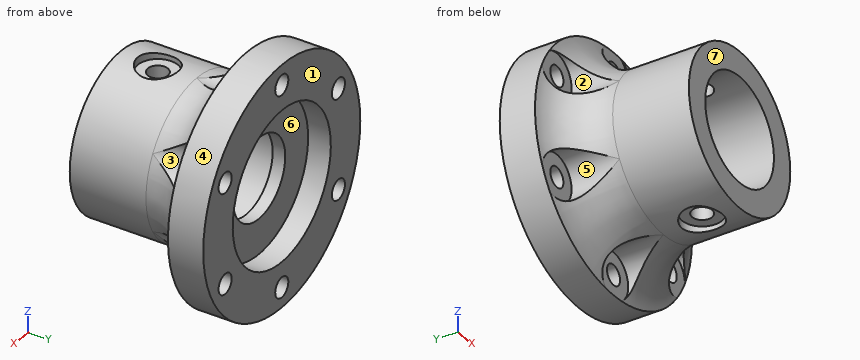
from build123d import *

# Parameters (mm, degrees)
SKETCH_1_R          = 15.5
SKETCH_1_R_2        = 10.5
EXTRUDE_1_DEPTH     = 25
SKETCH_3_R          = 24
EXTRUDE_2_DEPTH     = 7
FILLET_1_R          = 10
SKETCH_5_R          = 15
CUT_EXTRUDE_3_DEPTH = 4.5
SKETCH_6_R          = 8
CUT_EXTRUDE_4_DEPTH = 44.683520920365446
SKETCH_7_R          = 2.0000000000000018
SKETCH_7_R_2        = 2.0000000000000036
SKETCH_7_R_3        = 2.0000000000000004
SKETCH_7_R_4        = 2.0000000000000013
SKETCH_7_R_5        = 2.000000000000003
SKETCH_7_R_6        = 2
CUT_EXTRUDE_5_DEPTH = 47.64761515876246
CUT_EXTRUDE_START   = -7
SKETCH_8_R          = 4.500000000000001
SKETCH_8_R_2        = 4.500000000000002
SKETCH_8_R_3        = 4.5000000000000036
SKETCH_8_R_4        = 4.499999999999999
CUT_EXTRUDE_6_DEPTH = 10
SKETCH_9_R          = 2
CUT_EXTRUDE_7_DEPTH = 20
CUT_EXTRUDE_START_2 = -14
SKETCH_11_R         = 4
CUT_EXTRUDE_8_DEPTH = 40
CUT_EXTRUDE_START_3 = 54
SKETCH_12_R         = 4
CUT_EXTRUDE_9_DEPTH = 40


with BuildPart() as part:
    # Эскиз1 → Вытянуть1 (new body)
    with BuildSketch(Plane(origin=(0, 0, 0), x_dir=(1, 0, 0), z_dir=(0, 1, 0))):
        with Locations(Location((0, 0, 0), (0, 0, 270))):
            Circle(SKETCH_1_R)
        with Locations(Location((0, 0, 0), (0, 0, 270))):
            Circle(SKETCH_1_R_2, mode=Mode.SUBTRACT)
    extrude(amount=EXTRUDE_1_DEPTH)

    # Эскиз3 → Вытянуть2 (add)
    with BuildSketch(Plane(origin=(0, 25, 0), x_dir=(1, 0, 0), z_dir=(0, 1, 0))):
        with Locations(Location((0, 0, 0), (0, 0, 270))):
            Circle(SKETCH_3_R)
    extrude(amount=EXTRUDE_2_DEPTH)

    # Скругление1
    # the kernel refuses this fillet: 10 mm, written as the material it adds along each edge
    with BuildSketch(Plane(origin=(0, 25, 0), x_dir=(-1.8e-16, 0, 1), z_dir=(-1, 0, -1.8e-16))) as fillet_1_piece_1:
        with BuildLine():
            CenterArc((25.5, -9.886859966642819), FILLET_1_R, 98.62692655867845, 81.37307344132155)
            Line((15.5, -9.886859966642819), (15.3, -9.886859966642819))
            Line((15.3, -9.886859966642819), (15.3, 0))
            Line((15.3, 0), (15.5, 0.1999999999999993))
            ThreePointArc((15.5, 0.1999999999999993), (19.750000000000014, 0.1999999999999993), (23.970000000000034, 0.19773719933263223))
            Line((23.970000000000034, 0.19773719933263223), (24.000000000000032, -2.2027e-13))
        make_face()
    revolve(axis=Axis((0, 25, 0), (0, 1, 0)))

    # Эскиз5 → Вытянуть3 (cut)
    with BuildSketch(Plane(origin=(0, 32, 0), x_dir=(1, 0, 0), z_dir=(0, 1, 0))):
        with Locations(Location((0, 0, 0), (0, 0, 270))):
            Circle(SKETCH_5_R)
    extrude(amount=-CUT_EXTRUDE_3_DEPTH, mode=Mode.SUBTRACT)

    # Эскиз6 → Вытянуть4 (cut, through all)
    with BuildSketch(Plane(origin=(0, 27.5, 0), x_dir=(1, 0, 0), z_dir=(0, 1, 0))):
        with Locations(Location((0, 0, 0), (0, 0, 270))):
            Circle(SKETCH_6_R)
    extrude(amount=-CUT_EXTRUDE_4_DEPTH, mode=Mode.SUBTRACT)

    # Эскиз7 → Вытянуть5 (cut, through all)
    with BuildSketch(Plane(origin=(0, 32, 0), x_dir=(1, 0, 0), z_dir=(0, 1, 0))):
        with Locations(Location((0, -20, 0), (0, 0, 270))):
            Circle(SKETCH_7_R)
        with Locations(Location((-17.320508075688796, -9.999999999999961, 0), (0, 0, 270))):
            Circle(SKETCH_7_R_2)
        with Locations(Location((-17.320508075688732, 10.00000000000008, 0), (0, 0, 270))):
            Circle(SKETCH_7_R_3)
        with Locations(Location((1.3966e-13, 20, 0), (0, 0, 270))):
            Circle(SKETCH_7_R_4)
        with Locations(Location((17.32050807568886, 9.999999999999838, 0), (0, 0, 270))):
            Circle(SKETCH_7_R_5)
        with Locations(Location((17.320508075688657, -10.000000000000204, 0), (0, 0, 270))):
            Circle(SKETCH_7_R_6)
    extrude(amount=-CUT_EXTRUDE_5_DEPTH, mode=Mode.SUBTRACT)

    # Эскиз8 → Вытянуть6 (cut)
    with BuildSketch(Plane(origin=(0, 32, 0), x_dir=(1, 0, 0), z_dir=(0, 1, 0)).offset(CUT_EXTRUDE_START)):
        with Locations((0, -20)):
            Circle(SKETCH_8_R)
        with Locations((-17.320508075688796, -9.999999999999961)):
            Circle(SKETCH_8_R_2)
        with Locations((-17.320508075688732, 10.00000000000008)):
            Circle(SKETCH_8_R)
        with Locations((1.3966e-13, 20)):
            Circle(SKETCH_8_R)
        with Locations((17.32050807568886, 9.999999999999838)):
            Circle(SKETCH_8_R_3)
        with Locations((17.320508075688657, -10.000000000000204)):
            Circle(SKETCH_8_R_4)
    extrude(amount=-CUT_EXTRUDE_6_DEPTH, mode=Mode.SUBTRACT)

    # Эскиз9 → Вытянуть7 (cut, symmetric)
    with BuildSketch(Plane.XY):
        with Locations((0, 7.423633946327345)):
            Circle(SKETCH_9_R)
    extrude(amount=CUT_EXTRUDE_7_DEPTH, both=True, mode=Mode.SUBTRACT)

    # Эскиз11 → Вытянуть8 (cut)
    with BuildSketch(Plane.XY.offset(CUT_EXTRUDE_START_2)):
        with Locations((0, 7.423633946327345)):
            Circle(SKETCH_11_R)
    extrude(amount=-CUT_EXTRUDE_8_DEPTH, mode=Mode.SUBTRACT)

    # Эскиз12 → Вытянуть9 (cut)
    with BuildSketch(Plane.XY.offset(CUT_EXTRUDE_START_3)):
        with Locations((0, 7.423633946327345)):
            Circle(SKETCH_12_R)
    extrude(amount=-CUT_EXTRUDE_9_DEPTH, mode=Mode.SUBTRACT)


solid = part.part
Read the model definition and answer for the solid it produces. Units are mm, in the model's axes. Face numbers are marked on the shaded views. A direction names the side the tool comes from. Coordinates: 2 decimals unless noted, no trailing zeros. Loops run counter-clockwise (first coordinate to the right, second up) from the corner with the lowest first, then second, coordinate; pieces in that order, holes last. Notation, with made-up numbers: (65.5, 21) -> (124.5, 21) arc R16 cw to (124.5, 35) -> close; hole circle Ø4 at (1, 48.5). An arc over 180 degrees is marked (long way). Write item = value, one per line. Start each with the question number.
1) The mould has two halves that part along X. Classify the marked faces 1, 2, 3 and 4: pulls with the +X half, pulls with the -X half, needs draft (parallel to the pull), parting line crosses it, or undercut.
2) The part is cut by section B-B, the plane y = 19.5. Determine the outline of the cut face in (x, z).
3) For the marked faces 5, 6 and 7, determine the directions among +Z, -Z, +X, -X, +Y, -Y from which every point of the face is accessible in a straight line to the end or side of a thin tool.
4) Find the intervals of material crossed by L1, parallel to Z at x = 0, y = 16.5; L2, parallel to Z at x = -0.5, y = 28.5; L3, parallel to Y at x = -5, z = 11, in increasing order. Write a range as from..to.
5) The part is cut by section C-C, the plane x = -18. State how many separate pieces and enclosed holes the cut face has, plus the area to 3 significant figures.
6) The part is cut by section D-D, the plane y = 30. Determine the outline of the cut face in (x, z).
7) The part is cut by section A-A, the plane z = 0. Determine the outline of the cut face in (x, y), plus the area to 3 significant figures.
8) Given P1, Ø6.5, axis at x = 0, z = 20, coming from the -Y side; P2, Ø6.5, axis at x = 0, y = 7.42, coming from the -Z side; P3, Ø10, axis at x = -2, z = 7.5, coming from the +Y side; P4, Ø3, axis at x = -18.5, z = 11, coming from the +Y side, each flat-ended and moving along its own axis, determine where each tip first touches the part or whether it passes through.
Result:
q1.face_1 = needs draft
q1.face_2 = undercut
q1.face_3 = undercut
q1.face_4 = parting line crosses it
q2.outline = (-15.41, -5.92) arc R4.5 cw to (-12.84, -10.39) arc R16.51 ccw to (-2.58, -16.31) arc R4.5 cw to (2.58, -16.31) arc R16.51 ccw to (12.84, -10.39) arc R4.5 cw to (15.41, -5.92) arc R16.51 ccw to (15.41, 5.92) arc R4.5 cw to (12.84, 10.39) arc R16.51 ccw to (2.58, 16.31) arc R4.5 cw to (-2.58, 16.31) arc R16.51 ccw to (-12.84, 10.39) arc R4.5 cw to (-15.41, 5.92) arc R16.51 ccw to start; hole circle Ø21 at (0, 0)
q3.face_5 = -Y
q3.face_6 = +Y
q3.face_7 = +Z, -Z, +X, -X, -Y
q4.L1 = -15.5..-10.5, 10.5..15.5
q4.L2 = -23.99..-21.94, -18.06..-14.99, 14.99..18.06, 21.94..23.99
q4.L3 = 0..27.5
q5.separate_pieces = 3
q5.enclosed_holes = 0
q5.area = 203 mm²
q6.outline = circle Ø48 at (0, 0); hole circle Ø4 at (-17.32, -10); hole circle Ø4 at (-17.32, 10); hole circle Ø30 at (0, 0); hole circle Ø4 at (0, -20); hole circle Ø4 at (0, 20); hole circle Ø4 at (17.32, -10); hole circle Ø4 at (17.32, 10)
q7.outline = (-24, 25) arc R10 cw to (-15.5, 15.11) -> (-15.5, 0) -> (-10.5, 0) -> (-10.5, 25) -> (-8, 25) -> (-8, 27.5) -> (-15, 27.5) -> (-15, 32) -> (-24, 32) -> close; (8, 25) -> (10.5, 25) -> (10.5, 0) -> (15.5, 0) -> (15.5, 15.11) arc R10 cw to (24, 25) -> (24, 32) -> (15, 32) -> (15, 27.5) -> (8, 27.5) -> close
q7.area = 452 mm²
q8.P1 = 25
q8.P2 = -14
q8.P3 = 27.5
q8.P4 = 32
